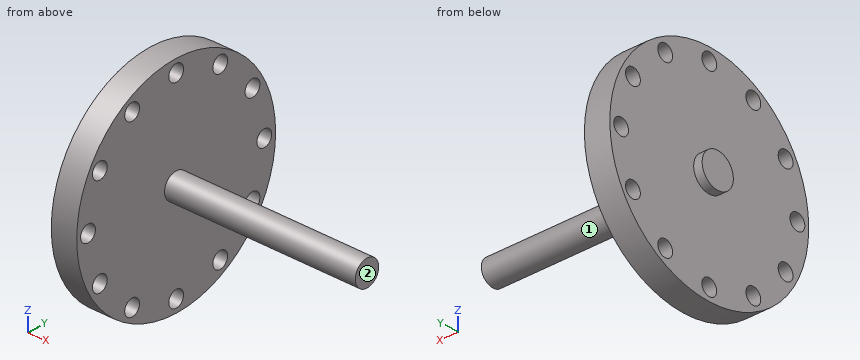
```python
from build123d import *

# Parameters (mm, degrees)
SKETCH_2_R           = 9.5
CUT_EXTRUDE_1_DEPTH  = 321.526909947
SKETCH_3_R           = 9.5
CUT_EXTRUDE_2_DEPTH  = 321.526909947
SKETCH_4_R           = 9.5
CUT_EXTRUDE_3_DEPTH  = 321.526909947
SKETCH_5_R           = 9.5
CUT_EXTRUDE_4_DEPTH  = 321.526909947
SKETCH_6_R           = 9.5
CUT_EXTRUDE_5_DEPTH  = 321.526909947
SKETCH_7_R           = 9.5
CUT_EXTRUDE_6_DEPTH  = 321.526909947
SKETCH_8_R           = 9.5
CUT_EXTRUDE_7_DEPTH  = 321.526909947
SKETCH_9_R           = 9.5
CUT_EXTRUDE_8_DEPTH  = 321.526909947
SKETCH_10_R          = 9.5
CUT_EXTRUDE_9_DEPTH  = 321.526909947
SKETCH_11_R          = 9.5
CUT_EXTRUDE_10_DEPTH = 321.526909947
SKETCH_12_R          = 9.5
CUT_EXTRUDE_11_DEPTH = 321.526909947
SKETCH_13_R          = 9.5
CUT_EXTRUDE_12_DEPTH = 321.526909947


with BuildPart() as part:
    # Эскиз1 → Повернуть1 (revolve)
    with BuildSketch(Plane.XY, mode=Mode.PRIVATE) as revolve_1_sk:
        Polygon((0, 0), (265, 0), (265, 15), (40, 15), (40, 127.5), (10, 127.5), (10, 20), (0, 20), align=None)
    revolve(revolve_1_sk.sketch.rotate(Axis((0, 0, 0), (1, 0, 0)), 90), axis=Axis((0, 0, 0), (1, 0, 0)))

    # Эскиз2 → Вырез-Вытянуть1 (cut, through all)
    with BuildSketch(Plane(origin=(0, 0, 0), x_dir=(0, 0, -1), z_dir=(1, 0, 0))):
        with Locations(Location((0, 113, 0), (0, 0, 180))):
            Circle(SKETCH_2_R)
    extrude(amount=CUT_EXTRUDE_1_DEPTH, mode=Mode.SUBTRACT)

    # Эскиз3 → Вырез-Вытянуть2 (cut, through all)
    with BuildSketch(Plane(origin=(0, 0, 0), x_dir=(0, 0, -1), z_dir=(1, 0, 0))):
        with Locations(Location((-56.5, 97.860870628, 0), (0, 0, 180))):
            Circle(SKETCH_3_R)
    extrude(amount=CUT_EXTRUDE_2_DEPTH, mode=Mode.SUBTRACT)

    # Эскиз4 → Вырез-Вытянуть3 (cut, through all)
    with BuildSketch(Plane(origin=(0, 0, 0), x_dir=(0, 0, -1), z_dir=(1, 0, 0))):
        with Locations(Location((-97.860870628, 56.5, 0), (0, 0, 180))):
            Circle(SKETCH_4_R)
    extrude(amount=CUT_EXTRUDE_3_DEPTH, mode=Mode.SUBTRACT)

    # Эскиз5 → Вырез-Вытянуть4 (cut, through all)
    with BuildSketch(Plane(origin=(0, 0, 0), x_dir=(0, 0, -1), z_dir=(1, 0, 0))):
        with Locations(Location((-113, 0, 0), (0, 0, 180))):
            Circle(SKETCH_5_R)
    extrude(amount=CUT_EXTRUDE_4_DEPTH, mode=Mode.SUBTRACT)

    # Эскиз6 → Вырез-Вытянуть5 (cut, through all)
    with BuildSketch(Plane(origin=(0, 0, 0), x_dir=(0, 0, -1), z_dir=(1, 0, 0))):
        with Locations(Location((-97.860870628, -56.5, 0), (0, 0, 180))):
            Circle(SKETCH_6_R)
    extrude(amount=CUT_EXTRUDE_5_DEPTH, mode=Mode.SUBTRACT)

    # Эскиз7 → Вырез-Вытянуть6 (cut, through all)
    with BuildSketch(Plane(origin=(0, 0, 0), x_dir=(0, 0, -1), z_dir=(1, 0, 0))):
        with Locations(Location((-56.5, -97.860870628, 0), (0, 0, 180))):
            Circle(SKETCH_7_R)
    extrude(amount=CUT_EXTRUDE_6_DEPTH, mode=Mode.SUBTRACT)

    # Эскиз8 → Вырез-Вытянуть7 (cut, through all)
    with BuildSketch(Plane(origin=(0, 0, 0), x_dir=(0, 0, -1), z_dir=(1, 0, 0))):
        with Locations(Location((0, -113, 0), (0, 0, 180))):
            Circle(SKETCH_8_R)
    extrude(amount=CUT_EXTRUDE_7_DEPTH, mode=Mode.SUBTRACT)

    # Эскиз9 → Вырез-Вытянуть8 (cut, through all)
    with BuildSketch(Plane(origin=(0, 0, 0), x_dir=(0, 0, -1), z_dir=(1, 0, 0))):
        with Locations(Location((56.5, -97.860870628, 0), (0, 0, 180))):
            Circle(SKETCH_9_R)
    extrude(amount=CUT_EXTRUDE_8_DEPTH, mode=Mode.SUBTRACT)

    # Эскиз10 → Вырез-Вытянуть9 (cut, through all)
    with BuildSketch(Plane(origin=(0, 0, 0), x_dir=(0, 0, -1), z_dir=(1, 0, 0))):
        with Locations(Location((97.860870628, -56.5, 0), (0, 0, 180))):
            Circle(SKETCH_10_R)
    extrude(amount=CUT_EXTRUDE_9_DEPTH, mode=Mode.SUBTRACT)

    # Эскиз11 → Вырез-Вытянуть10 (cut, through all)
    with BuildSketch(Plane(origin=(0, 0, 0), x_dir=(0, 0, -1), z_dir=(1, 0, 0))):
        with Locations(Location((113, 0, 0), (0, 0, 180))):
            Circle(SKETCH_11_R)
    extrude(amount=CUT_EXTRUDE_10_DEPTH, mode=Mode.SUBTRACT)

    # Эскиз12 → Вырез-Вытянуть11 (cut, through all)
    with BuildSketch(Plane(origin=(0, 0, 0), x_dir=(0, 0, -1), z_dir=(1, 0, 0))):
        with Locations(Location((97.860870628, 56.5, 0), (0, 0, 180))):
            Circle(SKETCH_12_R)
    extrude(amount=CUT_EXTRUDE_11_DEPTH, mode=Mode.SUBTRACT)

    # Эскиз13 → Вырез-Вытянуть12 (cut, through all)
    with BuildSketch(Plane(origin=(0, 0, 0), x_dir=(0, 0, -1), z_dir=(1, 0, 0))):
        with Locations(Location((56.5, 97.860870628, 0), (0, 0, 180))):
            Circle(SKETCH_13_R)
    extrude(amount=CUT_EXTRUDE_12_DEPTH, mode=Mode.SUBTRACT)


solid = part.part
```
The model under review builds one solid part; all positions refer to its coordinate system, in mm. Face numbers are marked on the shaded views. A direction names the side the tool comes from. Round coordinates to 2 decimals unless told otherwise and drop trailing zeros. Loops run counter-clockwise (first coordinate to the right, second up) from the corner with the lowest first, then second, coordinate; pieces in that order, holes last.
Item 1: Clearance check with flat-ended pins moving along their axes: pin 1 Ø15 at (y, z) = (0, -113) entering from +X; pin 2 Ø22 at (y, z) = (97.86, 56.5) entering from -X; pin 3 Ø5 at (y, z) = (45.5, -55) entering from +X; pin 4 Ø12 at (x, y) = (36.5, 56) entering from +Z. State where each tip first meets the part, or that it passes through.
Determined:
pin 1: passes through
pin 2: stops at x = 10
pin 3: stops at x = 40
pin 4: stops at z = 117.29
Item 2: Take a section at D-D (x = 239). Write out the cut boundary in (y, z).
Determined:
outline: circle Ø30 at (0, 0)
Item 3: Take a section at C-C (z = 111). Write out the cut boundary in (x, y), then the cut area to 3 significant figures.
Determined:
outline: (10, -62.73) - (40, -62.73) - (40, -9.29) - (10, -9.29) - close; (10, 9.29) - (40, 9.29) - (40, 62.73) - (10, 62.73) - close
area: 3,210 mm2
Item 4: Take a section at A-A (z = 0). Write out the cut boundary in (x, y).
Determined:
outline: (0, -20) - (10, -20) - (10, -103.5) - (40, -103.5) - (40, -15) - (265, -15) - (265, 15) - (40, 15) - (40, 103.5) - (10, 103.5) - (10, 20) - (0, 20) - close; (10, -127.5) - (40, -127.5) - (40, -122.5) - (10, -122.5) - close; (10, 122.5) - (40, 122.5) - (40, 127.5) - (10, 127.5) - close
Item 5: For the marked faces 1 and 2, list the 3-axis set-ups (+Z, -Z, +X, -X, +Y, -Y) from which the entire face can be reached by the end or side of a thin tool; tool diameter is ignored.
Determined:
face 1: +X
face 2: +Z, -Z, +X, +Y, -Y
Item 6: For line 1 (Y direction, x = 18.5, z = 0); line 2 (Y direction, x = 30.5, z = 56.5); line 3 (X direction, y = 45, z = -105), list the stretches that pass through material, from the lowest coordinate up.
Determined:
line 1: y = -127.5 to -122.5, -103.5 to 103.5, 122.5 to 127.5
line 2: y = -114.3 to -107.36, -88.36 to 88.36, 107.36 to 114.3
line 3: x = 10 to 40
